Input: part model. Units: mm. Frame: model coordinates. A direction names the side the tool comes from. Round coordinates to 2 decimals unless told otherwise and drop trailing zeros. Loops run counter-clockwise (first coordinate to the right, second up) from the corner with the lowest first, then second, coordinate; pieces in that order, holes last. Notation, with made-up numbers: M -32.75,-38 L -17.75,-38 A22 cw -17.75,-13 Z; hole C -20.75,-13.5 d11. An arc over 180 degrees is marked long. Put each result on its own line as item: value. Start each with the question number.
1) Reachability of faces 5 (the face through (50, 15, 7)), 6 (the face through (51, 50, 7)) from +Z, -Z, +X, -X, +Y, -Y: full face, straight path, thin tool, end or side. Return the list, or none.
2) Section A-A on z = 11.25. Output: boundary loops of the cut face in (x, y), plus the area to 3 significant figures.
3) Draft query along X for faces 1 (the face through (0, 25, 7)), 2 (the face through (30, 4, 7)), 3 (the face through (49, 25, 15)), 4 (the face through (32.406, 12.719, 7.605)). Return one class per face: +X half, -X half, draft (parallel to the pull), parting line (faces both ways), or undercut.
4) Section C-C on x = 20. Output: boundary loops of the cut face in (y, z).
5) Line query: probe 1 along X at (y, z) = (30, 3.5); probe 2 along Y at (x, z) = (80, 6.5); probe 3 along X at (y, z) = (33.5, 3). Output: solid intervals per line, ascending.
6) Section B-B on y = 30. Output: boundary loops of the cut face in (x, z), plus the area to 3 significant figures.
7) Pin query (flat end, axial travel): pin 1 (1 mm diameter, centred on x = 66, z = 8, fed in from -Y); pin 2 (4.5 mm diameter, centred on x = 52, z = 4.5, fed in from -Y); pin 3 (8 mm diameter, centred on x = 80, y = 30, fed in from -Z). Return the tip coordinate at first contact, or that it passes through.
8) Section D-D on x = 39. Output: boundary loops of the cut face in (y, z).
Solid Edge part; units mm, degrees
sketch "Sketch1" plane through (0, 0, 0) normal (0, 0, 1) x (1, 0, 0)
  line L0 (0, 0) -> (100, 0)
  line L1 (100, 0) -> (100, 50)
  line L2 (100, 50) -> (0, 50)
  line L3 (0, 50) -> (0, 0)
extrude "Protrusion1" add sketch "Sketch1" along normal blind 15
hole "Hole_1" at (80, 30, 15) direction (0, 0, -1) diameter 10 end through all
hole "Hole1" at (20, 30, 15) direction (0, 0, -1) diameter 10 end through all
sketch "Sketch2" plane through (50, 25, 0) normal (0, 0, -1) x (-1, 0, 0)
  line L0 (-20, -25) -> (-20, -10)
  line L1 (-20, -10) -> (20, -10)
  line L2 (20, -10) -> (20, -25)
  line L3 (-20, -25) -> (20, -25)
extrude "Cutout1" cut sketch "Sketch2" against normal through all
fillet "Round_1" radius 8 2 edges at (70, 15, 7.5) (30, 15, 7.5)
properties part number "1001"
Geometry results:
1. face 5: +Z, -Z, -Y
1. face 6: +Z, -Z, +X, -X, +Y
2. outline: M 0,0 L 30,0 L 30,7 A8 cw 38,15 L 62,15 A8 cw 70,7 L 70,0 L 100,0 L 100,50 L 0,50 Z; hole C 20,30 d10; hole C 80,30 d10
2. area: 4,270 mm²
3. face 1: -X half
3. face 2: undercut
3. face 3: draft
3. face 4: undercut
4. outline: M 0,0 L 25,0 L 25,15 L 0,15 Z; M 35,0 L 50,0 L 50,15 L 35,15 Z
5. probe 1: x = 0 to 15, 25 to 75, 85 to 100
5. probe 2: y = 0 to 25, 35 to 50
5. probe 3: x = 0 to 16.43, 23.57 to 76.43, 83.57 to 100
6. outline: M 0,0 L 15,0 L 15,15 L 0,15 Z; M 25,0 L 75,0 L 75,15 L 25,15 Z; M 85,0 L 100,0 L 100,15 L 85,15 Z
6. area: 1,200 mm²
7. pin 1: stops at y = 13.61
7. pin 2: stops at y = 15
7. pin 3: passes through
8. outline: M 15,0 L 50,0 L 50,15 L 15,15 Z
